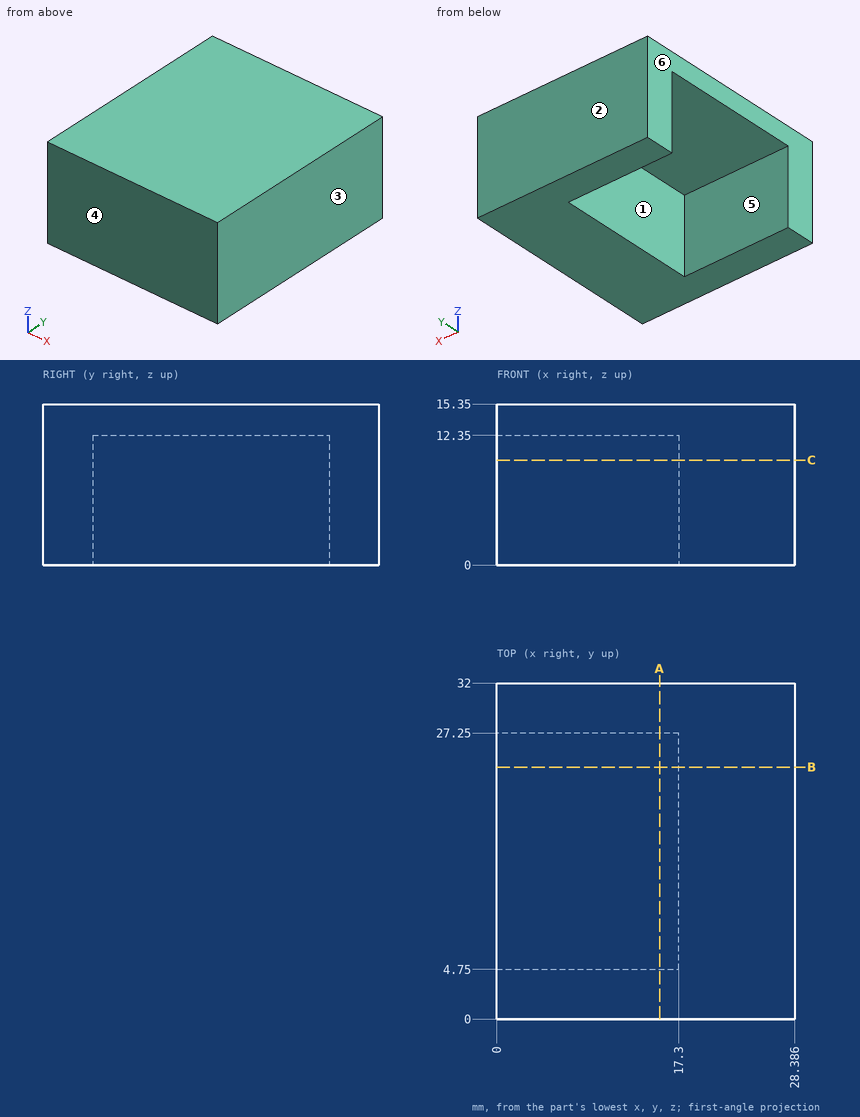
Design review of the part shown in the three views and the two pictorial views. Dimensions are in mm from the part's minimum x, y and z. A direction names the side the tool comes from. Round coordinates to 2 decimals unless told otherwise and drop trailing zeros. Loops run counter-clockwise (first coordinate to the right, second up) from the corner with the lowest first, then second, coordinate; pieces in that order, holes last.
Q1. Insertion check: pin 1 Ø5 at (x, y) = (9.5, 19) entering from -Z; pin 2 Ø6 at (y, z) = (11.5, 7.5) entering from -X. Each pin has a flat end and moves straight along its axis. Give the tip position at first contact, or say it passes through.
Result sheet:
pin 1: stops at z = 12.35
pin 2: stops at x = 17.3
Q2. Add section B-B on y = 24. Write out the cut boundary in (x, z), plus the area to 3 significant figures.
Result sheet:
outline: (0, 12.35) - (17.3, 12.35) - (17.3, 0) - (28.39, 0) - (28.39, 15.35) - (0, 15.35) - close
area: 222 mm2
Q3. To check wall thickness, follow line 1 along Y through (x, z) = (6.25, 2); line 2 along Z through (x, y) = (17, 6.5); line 3 along X through (y, z) = (8.5, 9.25). State the ranges of each line that lie inside material, in increasing order.
Result sheet:
line 1: y = 0 to 4.75, 27.25 to 32
line 2: z = 12.35 to 15.35
line 3: x = 17.3 to 28.39
Q4. Mouldability with a two-part tool opening along Y and no side actions: class the marked faces 1, 2, 3 and 4 as +Y half, -Y half, draft (parallel to the pull), parting line (faces both ways), or undercut.
Result sheet:
face 1: undercut
face 2: +Y half
face 3: draft
face 4: -Y half
Q5. Add section C-C on z = 10. Write out the cut boundary in (x, y), plus the area to 3 significant figures.
Result sheet:
outline: (0, 0) - (28.39, 0) - (28.39, 32) - (0, 32) - (0, 27.25) - (17.3, 27.25) - (17.3, 4.75) - (0, 4.75) - close
area: 519 mm2
Q6. Machinability: for the marked faces 5 and 6, which of the approach directions +Z, -Z, +X, -X, +Y, -Y give a long, thin tool a straight path to every point of the face, cutting with its end or side? Answer none if there is none.
Result sheet:
face 5: -Z, -X
face 6: +Z, -Z, -X, +Y, -Y
Q7. Add section A-A on x = 15.5. Write out the cut boundary in (y, z), plus the area to 3 significant figures.
Result sheet:
outline: (0, 0) - (4.75, 0) - (4.75, 12.35) - (27.25, 12.35) - (27.25, 0) - (32, 0) - (32, 15.35) - (0, 15.35) - close
area: 213 mm2
